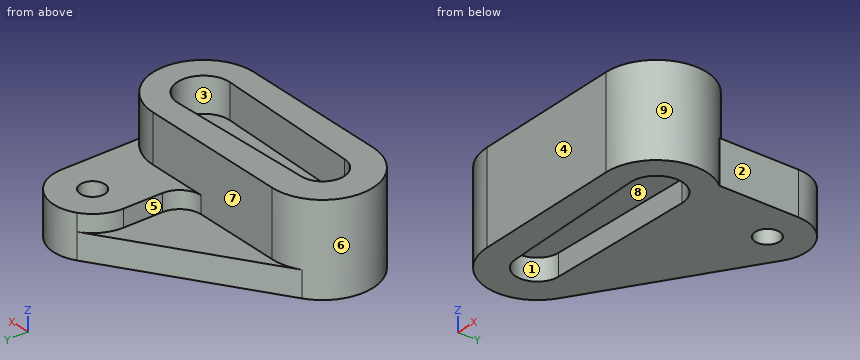
```python
from build123d import *

# Parameters (mm, degrees)
BOSS_EXTRUDE3_DEPTH      = 48
BOSS_EXTRUDE3_DEPTH_BACK = 15
BOSS_EXTRUDE4_DEPTH      = 24
BOSS_EXTRUDE5_DEPTH      = 15
BOSS_EXTRUDE5_DEPTH_BACK = 15
SKETCH2_6_R              = 8.5
BOSS_EXTRUDE6_DEPTH      = 3
BOSS_EXTRUDE6_DEPTH_BACK = 15


with BuildPart() as part:
    # Sketch2 → Boss-Extrude3 (new, two sides: drawn at the far end of the back side and taken through both)
    with BuildSketch(Plane.XY.offset(-BOSS_EXTRUDE3_DEPTH_BACK)):
        with BuildLine():
            ThreePointArc((45.747556009, -35), (80.747556009, 0), (45.747556009, 35))
            Line((45.747556009, 35), (3.747556009, 35))
            Line((3.747556009, 35), (-58.252443991, 35))
            ThreePointArc((-58.252443991, 35), (-93.252443991, 0), (-58.252443991, -35))
            Line((-58.252443991, -35), (45.747556009, -35))
        make_face()
        with BuildLine():
            ThreePointArc((45.22832524, -17.992509536), (63.747556009, 0), (45.22832524, 17.992509536))
            Line((45.22832524, 17.992509536), (-58.685136299, 14.993757947))
            ThreePointArc((-58.685136299, 14.993757947), (-73.252443991, 0), (-58.685136299, -14.993757947))
            Line((-58.685136299, -14.993757947), (45.22832524, -17.992509536))
        make_face(mode=Mode.SUBTRACT)
    extrude(amount=BOSS_EXTRUDE3_DEPTH + BOSS_EXTRUDE3_DEPTH_BACK)

    # Sketch2_5 → Boss-Extrude4 (add)
    with BuildSketch(Plane.XY):
        with BuildLine():
            Line((45.22832524, -17.992509536), (-58.685136299, -14.993757947))
            ThreePointArc((-58.685136299, -14.993757947), (-73.252443991, 0), (-58.685136299, 14.993757947))
            Line((-58.685136299, 14.993757947), (45.22832524, 17.992509536))
            ThreePointArc((45.22832524, 17.992509536), (63.747556009, 0), (45.22832524, -17.992509536))
        make_face()
    extrude(amount=BOSS_EXTRUDE4_DEPTH)

    # Sketch2_6 → Boss-Extrude5 (add, two sides: drawn at the far end of the back side and taken through both)
    with BuildSketch(Plane.XY.offset(-BOSS_EXTRUDE5_DEPTH_BACK)):
        with BuildLine():
            ThreePointArc((18.747556009, 50), (14.354157727, 39.393398282), (3.747556009, 35))
            Line((3.747556009, 35), (45.747556009, 35))
            ThreePointArc((45.747556009, 35), (60.672585141, 31.658229663), (72.747556009, 22.271057451))
            Line((72.747556009, 22.271057451), (72.747556009, 77))
            ThreePointArc((72.747556009, 77), (58.636796874, 100.724828132), (31.053669349, 99.651483281))
            ThreePointArc((31.053669349, 99.651483281), (22.022727876, 89.889240866), (18.747556009, 77))
            Line((18.747556009, 77), (18.747556009, 50))
        make_face()
        with Locations((45.747556009, 77)):
            Circle(SKETCH2_6_R, mode=Mode.SUBTRACT)
    extrude(amount=BOSS_EXTRUDE5_DEPTH + BOSS_EXTRUDE5_DEPTH_BACK)

    # Sketch2_7 → Boss-Extrude6 (add, two sides: drawn at the far end of the back side and taken through both)
    with BuildSketch(Plane.XY.offset(-BOSS_EXTRUDE6_DEPTH_BACK)):
        with BuildLine():
            ThreePointArc((-77.300074847, 29.363033883), (-68.184558925, 33.56118432), (-58.252443991, 35))
            Line((-58.252443991, 35), (3.747556009, 35))
            ThreePointArc((3.747556009, 35), (14.354157727, 39.393398282), (18.747556009, 50))
            Line((18.747556009, 50), (18.747556009, 77))
            ThreePointArc((18.747556009, 77), (22.022727876, 89.889240866), (31.053669349, 99.651483281))
            Line((31.053669349, 99.651483281), (-77.300074847, 29.363033883))
        make_face()
    extrude(amount=BOSS_EXTRUDE6_DEPTH + BOSS_EXTRUDE6_DEPTH_BACK)


solid = part.part
```
Could you check a few things on this model? Use its own coordinates, in mm. Face numbers are marked on the shaded views. A direction names the side the tool comes from. Coordinates: 2 decimals unless noted, no trailing zeros. Write each loop counter-clockwise with the first axis right and the second up, starting at its lowest first coordinate (ties: lowest second). Pieces come first, ordered by that corner, then holes. Notation, with made-up numbers: (-17, -3) -> (34, -3) arc R20 ccw to (34, 15) -> close; hole circle Ø1 at (23.5, 77.25). An arc over 180 degrees is marked (long way). Return JSON: item names as keys, results as strings.
(1) Imagine slicing it at B-B, the plane y = 0. Please give me the cut outline in (x, z), then the cut area to 3 significant figures.
Numbers:
{"outline": "(-93.25, -15) -> (-73.25, -15) -> (-73.25, 0) -> (63.75, 0) -> (63.75, -15) -> (80.75, -15) -> (80.75, 48) -> (63.75, 48) -> (63.75, 24) -> (-73.25, 24) -> (-73.25, 48) -> (-93.25, 48) -> close", "area": "5,620 mm2"}
(2) Imagine slicing it at C-C, the plane x = -12. Please give me the cut outline in (y, z).
Numbers:
{"outline": "(-35, -15) -> (-16.34, -15) -> (-16.34, 0) -> (16.34, 0) -> (16.34, -15) -> (71.72, -15) -> (71.72, 3) -> (35, 3) -> (35, 48) -> (16.34, 48) -> (16.34, 24) -> (-16.34, 24) -> (-16.34, 48) -> (-35, 48) -> close"}
(3) I need wall thicknesses on L1, parallel to Y at x = 42.5, z = 26; L2, parallel to Z at x = -26.5, y = 9; L3, parallel to Y at x = 38, z = 8. Which ranges of each line are inside material? Lowest first, please.
Numbers:
{"L1": "y = -35 to -17.91, 17.91 to 35", "L2": "z = 0 to 24", "L3": "y = -35 to 73.5, 80.5 to 102.86"}
(4) I'm going to push flat-ended pins straight in: pin 1 (8 mm diameter, centred on y = 21.5, z = -4, fed in from +X); pin 2 (3 mm diameter, centred on y = -0.5, z = 26, fed in from -X); pin 3 (1 mm diameter, centred on x = 48, z = 20.5, fed in from +Y); pin 4 (15.5 mm diameter, centred on x = 45.75, y = 77, fed in from -Z). Where does each tip first touch, or does it pass through?
Numbers:
{"pin 1": "stops at x = 76.06", "pin 2": "stops at x = -93.25", "pin 3": "stops at y = 34.96", "pin 4": "passes through"}
(5) Which directions (+Z, -Z, +X, -X, +Y, -Y) give clear straight access to the entire face, cutting with the end or side of a thin tool? Please do the marked faces 1, 2, 3, 4 and 5.
Numbers:
{"face 1": "-Z", "face 2": "+Z, -Z, +X, +Y", "face 3": "+Z", "face 4": "+Z, -Z, +X, -X, -Y", "face 5": "+Z, -X, +Y"}
(6) We'd pull the mould along X, two halves only. Please class the marked faces 6, 7, 8 and 9: +X half, -X half, draft (parallel to the pull), parting line (faces both ways), or undercut.
Numbers:
{"face 6": "-X half", "face 7": "draft", "face 8": "undercut", "face 9": "+X half"}
(7) Imagine slicing it at A-A, the plane z = 28. Please give me the cut outline in (x, y), then the cut area to 3 significant figures.
Numbers:
{"outline": "(-58.25, -35) -> (45.75, -35) arc R35 ccw to (45.75, 35) -> (-58.25, 35) arc R35 ccw to start; hole (-58.69, -14.99) -> (45.23, -17.99) arc R18 ccw (long way) to (45.23, 17.99) -> (-58.69, 14.99) arc R15 ccw to start", "area": "6,830 mm2"}
(8) Imagine slicing it at D-D, the plane z = 9. Please give me the cut outline in (x, y).
Numbers:
{"outline": "(-58.25, -35) -> (45.75, -35) arc R35 ccw to (72.75, 22.27) -> (72.75, 77) arc R27 ccw to (18.75, 77) -> (18.75, 50) arc R15 cw to (3.75, 35) -> (-58.25, 35) arc R35 ccw to start; hole circle Ø17 at (45.75, 77)"}
